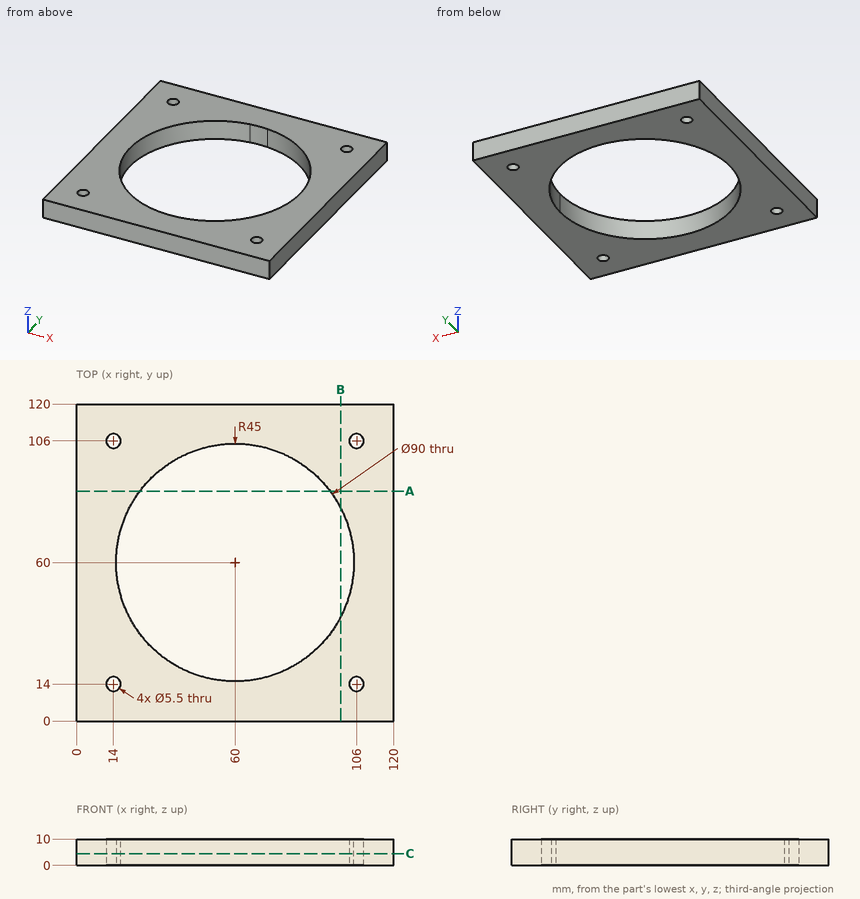
Can you work these out from the drawing? Everything is in mm from the part's minimum corner. Coordinates: 2 decimals unless noted, no trailing zeros. Write each loop counter-clockwise with the first axis right and the second up, starting at its lowest first coordinate (ties: lowest second). Pieces come first, ordered by that corner, then holes. Notation, with made-up numbers: (-11, -13) -> (4, -13) arc R22 cw to (4, 1) -> close; hole circle Ø10 at (-1.75, 11.5). An arc over 180 degrees is marked (long way). Write item = value, one per line.
(1) Imagine slicing it at C-C (z = 4.5). Please give me the cut outline in (x, y), and give its area (3 significant figures).
Verdict:
outline = (0, 0) -> (120, 0) -> (120, 120) -> (0, 120) -> close; hole circle Ø5.5 at (14, 14); hole circle Ø5.5 at (14, 106); hole (55.32, 104.76) arc R45 ccw (long way) to (64.68, 104.76) arc R45 ccw to start; hole circle Ø5.5 at (106, 14); hole circle Ø5.5 at (106, 106)
area = 7,940 mm^2
(2) If I drill on probe 1 along Y at (x, z) = (14, 6); probe 2 along Y at (x, z) = (60, 4.5), over which ranges is the centre line in solid material (lowest first)?
Verdict:
probe_1 = 0 to 11.25, 16.75 to 103.25, 108.75 to 120
probe_2 = 0 to 15, 105 to 120
(3) Imagine slicing it at A-A (y = 87). Please give me the cut outline in (x, z).
Verdict:
outline = (0, 0) -> (24, 0) -> (24, 10) -> (0, 10) -> close; (96, 0) -> (120, 0) -> (120, 10) -> (96, 10) -> close
(4) Imagine slicing it at B-B (x = 100). Please give me the cut outline in (y, z).
Verdict:
outline = (0, 0) -> (39.38, 0) -> (39.38, 10) -> (0, 10) -> close; (80.62, 0) -> (120, 0) -> (120, 10) -> (80.62, 10) -> close
